```python
from build123d import *
from build123d import SkipClean  # not in build123d's __all__

# Parameters (mm, degrees)
F0_W      = 131
F0_H      = 155.25
F0_R      = 5
F0_R_2    = 10
F1_DEPTH  = 12.7
F2_DEPTH  = 150
F3_R      = 4.7625
F4_DEPTH  = 167.951
F6_DEPTH  = 55
F9_W      = 46.4503765106
F9_H      = 23.6088857055
F10_DEPTH = 100.6187200546
F12_DEPTH = 150.001
F14_DEPTH = 89.0000760555
F15_R     = 18.8692896997
F16_DEPTH = 210.4837932836
F18_W     = 28.0103459954
F18_H     = 33.3821959794
F19_DEPTH = 57.4413500726
F23_DEPTH = 37.3063087463
F25_DEPTH = 262.8513174901
F26_W     = 130
F26_H     = 33
F27_DEPTH = 25
F28_DEPTH = 47.1665114164
F29_W     = 130
F29_H     = 16.5
F30_DEPTH = 374.0004003048


with BuildPart() as f1:
    # F0 (on Front) → F1 (new body)
    with BuildSketch(Plane.XZ):
        with Locations((0, 77.625)):
            Rectangle(F0_W, F0_H)
        with Locations((-32.75, 57)):
            Circle(F0_R, mode=Mode.SUBTRACT)
        with Locations((32.75, 57)):
            Circle(F0_R, mode=Mode.SUBTRACT)
        with Locations((0, 89.75)):
            Circle(F0_R_2, mode=Mode.SUBTRACT)
        with Locations((-32.75, 122.5)):
            Circle(F0_R, mode=Mode.SUBTRACT)
        with Locations((32.75, 122.5)):
            Circle(F0_R, mode=Mode.SUBTRACT)
    extrude(amount=-F1_DEPTH)

    # F0 (on Front) → F2 (join)
    with BuildSketch(Plane.XZ):
        Polygon((89.5, 0), (65.5, 0), (-65.5, 0), (-65.5, -12.7), (89.5, -12.7), align=None)
    extrude(amount=-F2_DEPTH)

    # F3 (on face) → F4 (cut, through all)
    with BuildSketch(Plane(origin=(0, 0, -12.7), x_dir=(1, 0, 0), z_dir=(0, 0, -1))):
        with Locations((-40, -55.7)):
            Circle(F3_R)
        with Locations((-40, -118.2)):
            Circle(F3_R)
        with Locations((64, -118.2)):
            Circle(F3_R)
        with Locations((64, -55.7)):
            Circle(F3_R)
    extrude(amount=-F4_DEPTH, mode=Mode.SUBTRACT)

    # F5 (on face) → F6 (join)
    with BuildSketch(Plane.XZ):
        Polygon((76.5, -12.7), (-63.5, -12.7), (-44.9285714286, -100.7630571853), align=None)
    extrude(amount=-F6_DEPTH)

    # F7 (on face) → F8 (revolve)
    with BuildSketch(Plane(origin=(32.4031609217, 0, -44.6801379177), x_dir=(0.8095238095, 0, 0.5870870479), z_dir=(0.5870870479, 0, -0.8095238095))):
        Polygon((18.2698592544, -37.5), (54.4725659202, -37.5), (54.4725659202, -30), (-45.5274340798, -30), (-45.5274340798, -37.5), align=None)
    revolve(axis=Axis((36.0238095238, 55, -42.0543523951), (-0.8095238095, 0, -0.5870870479)))

    # F9 (on face) → F10 (cut)
    with BuildSketch(Plane.YZ.offset(89.5)):
        with Locations((57.3695674539, 11.8044428527)):
            Rectangle(F9_W, F9_H)
    extrude(amount=-F10_DEPTH, mode=Mode.SUBTRACT)

    # F11 (on Front) → F12 (cut, through all)
    with BuildSketch(Plane.XZ):
        Polygon((-55.6169226766, -72.8361010551), (-44.6262694895, -72.8361010551), (-44.6262694895, -12.6905664802), (-63.8953074813, -12.6905664802), (-63.8953074813, -72.8361010551), align=None)
        Polygon((-4.5890193433, -104.113265872), (-4.5890193433, -72.8361010551), (-44.6262694895, -72.8361010551), (-55.6169226766, -72.8361010551), (-55.6169226766, -104.113265872), align=None)
    extrude(amount=-F12_DEPTH, mode=Mode.SUBTRACT)

    # F13 (on face) → F14 (cut)
    with BuildSketch(Plane(origin=(0, 55, 0), x_dir=(-1, 0, 0), z_dir=(0, 1, 0))):
        Polygon((76.3912552581, -71.6465198879), (44.6262694895, -60.2878452083), (44.6262694895, -72.8361010551), (6.4205920826, -72.8361010551), (4.4523809524, -71.4087047902), (-10.0519139283, -91.4084170785), (37.2047263411, -125.6801223738), align=None)
        Polygon((44.6262694895, -60.2878452083), (19.1295571499, -51.1706095521), (14.7264042907, -57.2420381235), (4.4523809524, -71.4087047902), (6.4205920826, -72.8361010551), (44.6262694895, -72.8361010551), align=None)
    extrude(amount=-F14_DEPTH, mode=Mode.SUBTRACT)

    # F15 (on face) → F16 (cut, through all)
    with BuildSketch(Plane(origin=(-36.8555418741, 0, -26.7285668724), x_dir=(0, -1, 0), z_dir=(-0.8095238095, 0, -0.5870870479))):
        with Locations((-55, -55.1931115454)):
            Circle(F15_R)
        with BuildLine():
            ThreePointArc((-37.5, -55.1931115454), (-67.3743686708, -67.5674802162), (-55, -37.6931115454))
            Line((-55, -37.6931115454), (-55, -55.1931115454))
            Line((-55, -55.1931115454), (-37.5, -55.1931115454))
        make_face(mode=Mode.SUBTRACT)
        with BuildLine():
            Line((-55, -55.1931115454), (-55, -37.6931115454))
            ThreePointArc((-55, -37.6931115454), (-67.3743686708, -67.5674802162), (-37.5, -55.1931115454))
            Line((-37.5, -55.1931115454), (-55, -55.1931115454))
        make_face()
    with SkipClean():  # cleaning this boolean's faces spoils the solid; the shape is the same uncleaned
        extrude(amount=-F16_DEPTH, mode=Mode.SUBTRACT)

    # F18 (on offset) → F19 (cut)
    with BuildSketch(Plane(origin=(0, 0, -69.7121929049), x_dir=(1, 0, 0), z_dir=(0, 0, -1))):
        with Locations((-40.2482412755, -55.8588486165)):
            Rectangle(F18_W, F18_H)
    with SkipClean():  # cleaning this boolean's faces spoils the solid; the shape is the same uncleaned
        extrude(amount=-F19_DEPTH, mode=Mode.SUBTRACT)

    # F22 (on offset) → F23 (join)
    with BuildSketch(Plane(origin=(0, 66.3563400507, 0), x_dir=(-1, 0, 0), z_dir=(0, 1, 0))):
        Polygon((-19.5, -25.368578732), (9.2864632607, -47.1396760544), (25.5, -47.1396760544), (25.5, -10.8354373375), (-19.5, -10.8354373375), align=None)
    with SkipClean():  # cleaning this boolean's faces spoils the solid; the shape is the same uncleaned
        extrude(amount=-F23_DEPTH)

    # F24 (on offset) → F25 (cut, through all)
    with BuildSketch(Plane(origin=(0, 0, -107.6003174901), x_dir=(1, 0, 0), z_dir=(0, 0, -1))):
        Polygon((105.054743588, -47.2050309181), (-70.2532827854, -47.2050309181), (-70.2532827854, -164.4858419895), (108.5324063897, -164.4858419895), align=None)
    extrude(amount=-F25_DEPTH, mode=Mode.SUBTRACT)

    # F26 (on Front) → F27 (join)
    with BuildSketch(Plane.XZ):
        with Locations((0.4943662184, -6)):
            Rectangle(F26_W, F26_H)
    extrude(amount=F27_DEPTH)

    # F28 (add): a face of the model
    f28_faces = [f1.faces().sort_by_distance(p)[0] for p in [
        (-54.5656671683, 0, -17.5954279167),
    ]]
    extrude(f28_faces, amount=F28_DEPTH)

    # F29 (on face) → F30 (cut)
    with BuildSketch(Plane.XZ.offset(25)):
        Polygon((102.4388783057, -90.8307954669), (102.4388783057, -6), (65.4943662184, -6), (65.4943662184, -22.5), (-64.5056337816, -22.5), (-64.5056337816, -6), (-95.0750373681, -6), (-96.5073853731, -90.8307954669), align=None)
        with Locations((0.4943662184, -14.25)):
            Rectangle(F29_W, F29_H)
    extrude(amount=-F30_DEPTH, mode=Mode.SUBTRACT)


solid = f1.part
```
CAD build for the part. Positions are in the model's coordinates, mm. A direction names the side the tool comes from. Round coordinates to 2 decimals unless told otherwise and drop trailing zeros. Order: outer loops, then holes, each group sorted by start corner. A loop starts at its lowest first (then second) coordinate and runs counter-clockwise, first axis right, second up. Notation, with made-up numbers: (-28, -7.5) -> (-8, -7.5) arc R27 ccw to (-8, 26.5) -> close; hole circle Ø10 at (-19.5, 45). An arc over 180 degrees is marked (long way). One line per question, with ' | ' between items.
Q1. Slice it at D-D (z = 89.75). Write the cut outline in (x, y).
Completed:
outline: (-65.5, 0) -> (-10, 0) -> (-10, 12.7) -> (-65.5, 12.7) -> close; (10, 0) -> (65.5, 0) -> (65.5, 12.7) -> (10, 12.7) -> close
Q2. Probe probe 1 along Z at (x, y) = (-32.75, 5.25); probe 2 along Z at (x, y) = (32, 2); probe 3 along Y at (x, z) = (17, 82). List the from-to ranges inside material, lowest first.
Completed:
probe 1: z = -6 to 52, 62 to 117.5, 127.5 to 155.25 | probe 2: z = -6 to 52.06, 61.94 to 117.56, 127.44 to 155.25 | probe 3: y = 0 to 12.7
Q3. Slice it at C-C (x = 0). Write the cut outline in (y, z), then the cut area to 3 significant figures.
Completed:
outline: (-25, -6) -> (47.21, -6) -> (47.21, 0) -> (12.7, 0) -> (12.7, 79.75) -> (0, 79.75) -> (0, 10.5) -> (-25, 10.5) -> close; (0, 99.75) -> (12.7, 99.75) -> (12.7, 155.25) -> (0, 155.25) -> close | area: 2,410 mm^2
Q4. Slice it at B-B (z = 60). Write the cut outline in (x, y), then the cut area to 3 significant figures.
Completed:
outline: (-65.5, 0) -> (-36.75, 0) -> (-36.75, 12.7) -> (-65.5, 12.7) -> close; (-28.75, 0) -> (28.75, 0) -> (28.75, 12.7) -> (-28.75, 12.7) -> close; (36.75, 0) -> (65.5, 0) -> (65.5, 12.7) -> (36.75, 12.7) -> close | area: 1,460 mm^2
Q5. Which spindle directions (+Z, -Z, +X, -X, +Y, -Y) get a long thin tool onto all of the face, cutting with end or side? Do faces 4 (the cylindrical face through (-36.435, 6.261, 60.379)), 5 (the flat face through (65.494, -12, 2)), 6 (the flat face through (-1, 12.7, 79)), 7 (the flat face through (0, -12, 10.5)), 8 (the flat face through (-64.506, -13, 2)). Say none if no direction does.
Completed:
face 4: +Y, -Y | face 5: +Z, -Z, +X, -Y | face 6: +Z, +X, -X, +Y | face 7: +Z, +X, -X, -Y | face 8: +Z, -Z, -X, -Y
Q6. Drop flat-ended pins along their axis: pin 1 (1 mm diameter, centred on x = -11, z = 57, fed in from -Y); pin 2 (16 mm diameter, centred on x = -32.75, z = 57, fed in from +Y); pin 3 (8 mm diameter, centred on y = 6.5, z = 130.5, fed in from +X); pin 4 (16 mm diameter, centred on x = 0, z = 89.75, fed in from -Y). Give the stop position or say it passes through.
Completed:
pin 1: stops at y = 0 | pin 2: stops at y = 12.7 | pin 3: stops at x = 65.5 | pin 4: passes through
Q7. Two-plate mould, pull along Z, no slides. Class faces 1 (the flat face through (11, 0, 94)), 2 (the cylindrical face through (29.065, 6.261, 60.379)), 3 (the flat face through (-1, 6, 155.25)): released by +Z, released by -Z, zero draft, split by the parting line, or undercut.
Completed:
face 1: zero draft | face 2: undercut | face 3: released by +Z
Q8. Slice it at A-A (x = -32.75). Write the cut outline in (y, z), then the cut area to 3 significant figures.
Completed:
outline: (-25, -6) -> (47.21, -6) -> (47.21, 0) -> (12.7, 0) -> (12.7, 52) -> (0, 52) -> (0, 10.5) -> (-25, 10.5) -> close; (0, 62) -> (12.7, 62) -> (12.7, 117.5) -> (0, 117.5) -> close; (0, 127.5) -> (12.7, 127.5) -> (12.7, 155.25) -> (0, 155.25) -> close | area: 2,410 mm^2
